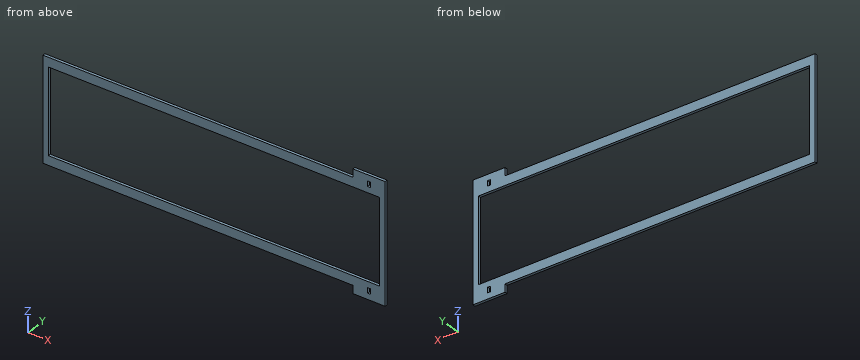
```python
from build123d import *

# Parameters (mm, degrees)
SKETCH1_W           = 3.175
SKETCH1_H           = 6.35
SKETCH1_W_2         = 393.7
SKETCH1_H_2         = 101.6
BOSS_EXTRUDE1_DEPTH = 1.5875


with BuildPart() as part:
    # Sketch1 → Boss-Extrude1 (new body, symmetric)
    with BuildSketch(Plane(origin=(0, 0, 0), x_dir=(1, 0, 0), z_dir=(0, 1, 0))):
        Polygon((203.2, 71.4375), (165.1, 71.4375), (165.1, 61.9125), (-203.2, 61.9125), (-203.2, 50.8), (-203.2, -50.8), (-203.2, -61.9125), (165.1, -61.9125), (165.1, -71.4375), (203.2, -71.4375), (203.2, -50.8), (203.2, 50.8), align=None)
        with Locations((184.15, -61.11875)):
            Rectangle(SKETCH1_W, SKETCH1_H, mode=Mode.SUBTRACT)
        Rectangle(SKETCH1_W_2, SKETCH1_H_2, mode=Mode.SUBTRACT)
        with Locations((184.15, 61.11875)):
            Rectangle(SKETCH1_W, SKETCH1_H, mode=Mode.SUBTRACT)
    extrude(amount=BOSS_EXTRUDE1_DEPTH, both=True)


solid = part.part
```
Here's how the part is built. I have some questions about the finished solid (model axes, mm). Round coordinates to 2 decimals unless told otherwise and drop trailing zeros. Order: outer loops, then holes, each group sorted by start corner. A loop starts at its lowest first (then second) coordinate and runs counter-clockwise, first axis right, second up. Notation, with made-up numbers: (88.25, 82.25) -> (145.25, 82.25) arc R21 cw to (145.25, 101.25) -> close; hole circle Ø11 at (-23, 1.25). An arc over 180 degrees is marked (long way). Use a Markdown table: item, result. Add a question column.
(1) Suppose I cut it at B-B, the plane z = 19.5. Please give me the cut outline in (x, y), and give its area (3 significant figures).
(2) For pin 1 Ø1 at (x, y) = (-29.5, 1) entering from -Z; pin 2 Ø1.6 at (x, y) = (-51, 0) entering from +Z, each with a flat end and sliding along its axis, tell me the tip position at first contact or that it passes through.
(3) I need wall thicknesses on line 1 along X through (y, z) = (0, 26.5); line 2 along Z through (x, y) = (-186, 0); line 3 along X through (y, z) = (-0.4, -62). Which ranges of each line are inside material? Lowest first, please.
(4) Suppose I cut it at C-C, the plane y = -0.8. Please give me the cut outline in (x, z), and give its area (3 significant figures).
(5) Suppose I cut it at A-A, the plane x = -7. Please give me the cut outline in (y, z), and give its area (3 significant figures).
Verdict:
| question | item | result |
|---|---|---|
| 1 | outline | (-203.2, -1.59) -> (-196.85, -1.59) -> (-196.85, 1.59) -> (-203.2, 1.59) -> close; (196.85, -1.59) -> (203.2, -1.59) -> (203.2, 1.59) -> (196.85, 1.59) -> close |
| 1 | area | 40.3 mm2 |
| 2 | pin 1 | z = -61.91 |
| 2 | pin 2 | z = 61.91 |
| 3 | line 1 | -203.2 to -196.85, 196.85 to 203.2 |
| 3 | line 2 | -61.91 to -50.8, 50.8 to 61.91 |
| 3 | line 3 | 165.1 to 182.56, 185.74 to 203.2 |
| 4 | outline | (-203.2, -61.91) -> (165.1, -61.91) -> (165.1, -71.44) -> (203.2, -71.44) -> (203.2, 71.44) -> (165.1, 71.44) -> (165.1, 61.91) -> (-203.2, 61.91) -> close; hole (-196.85, -50.8) -> (196.85, -50.8) -> (196.85, 50.8) -> (-196.85, 50.8) -> close; hole (182.56, -64.29) -> (185.74, -64.29) -> (185.74, -57.94) -> (182.56, -57.94) -> close; hole (182.56, 57.94) -> (185.74, 57.94) -> (185.74, 64.29) -> (182.56, 64.29) -> close |
| 4 | area | 11,000 mm2 |
| 5 | outline | (-1.59, -61.91) -> (1.59, -61.91) -> (1.59, -50.8) -> (-1.59, -50.8) -> close; (-1.59, 50.8) -> (1.59, 50.8) -> (1.59, 61.91) -> (-1.59, 61.91) -> close |
| 5 | area | 70.6 mm2 |
